For this review, take the finished solid that the model builds, in its own axes (mm). Give positions to 0.01 mm unless a question says otherwise; leave off trailing zeros.
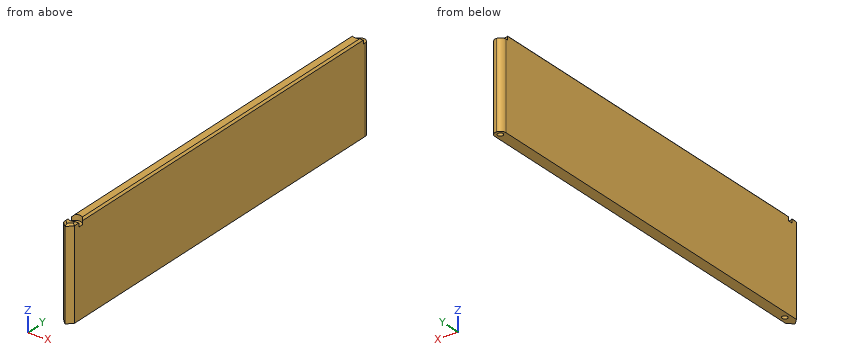
```python
from build123d import *

# Parameters (mm, degrees)
F0_W     = 438
F0_H     = 100
F1_DEPTH = 12
F2_R     = 3
F3_DEPTH = 120
F4_START = 94
F2_R_2   = 6.5
F4_DEPTH = 6
F5_SIZE  = 5.99999
F6_SIZE  = 2
F7_R     = 5.99999


# Not quite as in the source:
# - a fillet or chamfer is up to 0.001 mm smaller than in the source, because OpenCascade refuses the exact size


with BuildPart() as f1:
    # F0 (on Right) → F1 (new body)
    with BuildSketch(Plane.YZ):
        with Locations((-219, 50)):
            Rectangle(F0_W, F0_H)
    extrude(amount=F1_DEPTH)

    # F2 (on Top) → F3 (cut)
    with BuildSketch(Plane.XY):
        with Locations((6, -422.9574446679)):
            Circle(F2_R)
        with Locations((6, -6)):
            Circle(F2_R)
    extrude(amount=F3_DEPTH, mode=Mode.SUBTRACT)

    # F2 (on Top) → F4 (cut)
    with BuildSketch(Plane.XY.offset(F4_START)):
        with Locations((6, -6)):
            Circle(F2_R_2)
        with Locations((6, -6)):
            Circle(F2_R, mode=Mode.SUBTRACT)
        with Locations((6, -422.9574446679)):
            Circle(F2_R_2)
        with Locations((6, -422.9574446679)):
            Circle(F2_R, mode=Mode.SUBTRACT)
    extrude(amount=F4_DEPTH, mode=Mode.SUBTRACT)

    # F5 (size 6 in the source; OpenCascade refuses exactly that, so slightly less here)
    f5_edges = [f1.edges().sort_by_distance(p)[0] for p in [
        (12, -438, 50),
        (0, -438, 50),
    ]]
    chamfer(f5_edges, length=F5_SIZE)

    # F6 (call 1 of 4: OpenCascade refuses the feature's edges together)
    f6_edges = [f1.edges().sort_by_distance(p)[0] for p in [
        (12, -428.728727, 100),
        (9.000005, -435.000005, 100),
    ]]
    chamfer(f6_edges, length=F6_SIZE)

    # F6#2 (call 2 of 4)
    f6_2_edges = [f1.edges().sort_by_distance(p)[0] for p in [
        (0, -428.728727, 100),
        (2.999995, -435.000005, 100),
    ]]
    chamfer(f6_2_edges, length=F6_SIZE)

    # F6#3 (call 3 of 4)
    f6_3_edges = [f1.edges().sort_by_distance(p)[0] for p in [
        (12, -214.478722, 100),
    ]]
    chamfer(f6_3_edges, length=F6_SIZE)

    # F6#4 (call 4 of 4)
    f6_4_edges = [f1.edges().sort_by_distance(p)[0] for p in [
        (0, -214.478722, 100),
    ]]
    chamfer(f6_4_edges, length=F6_SIZE)

    # F7 (radius 6 in the source; OpenCascade refuses exactly that, so slightly less here)
    f7_edges = [f1.edges().sort_by_distance(p)[0] for p in [
        (12, 0, 50),
        (0, 0, 50),
    ]]
    fillet(f7_edges, radius=F7_R)


solid = f1.part
```
Q1. For pin 1 Ø3.5 at (x, y) = (4.5, -424.5) entering from +Z; pin 2 Ø1 at (x, z) = (7, 44.5) entering from -Y; pin 3 Ø2 at (x, z) = (8.5, 11.5) entering from +Y, all flat-tipped, find the tip position at first contact; note any pin that passes through.
Answers:
pin 1: stops at z = 94
pin 2: stops at y = -437.5
pin 3: stops at y = -0.19
Q2. Consider section A-A on z = 68. Count the separate pieces of the cut face and the enclosed holes in it, plus the area to 3 significant figures.
Answers:
separate pieces: 1
enclosed holes: 2
area: 5,150 mm2
Q3. For probe 1 along Y at (x, z) = (4, 56); probe 2 along Y at (x, z) = (6.5, 89); probe 3 along Z at (x, y) = (1.5, -40), list the stretches that pass through material, from the lowest coordinate up.
Answers:
probe 1: y = -436 to -425.19, -420.72 to -8.24, -3.76 to -0.34
probe 2: y = -437.5 to -425.92, -420 to -8.96, -3.04 to -0.02
probe 3: z = 0 to 99.5
